Part model, mm, in its own coordinate system. A direction names the side the tool comes from. Round coordinates to 2 decimals unless told otherwise and drop trailing zeros. Order: outer loops, then holes, each group sorted by start corner. A loop starts at its lowest first (then second) coordinate and runs counter-clockwise, first axis right, second up. Notation, with made-up numbers: (69, -32) - (90, -32) arc R20 cw to (90, -28) - close; hole circle Ø8 at (4, 62.25). An arc over 180 degrees is marked (long way). Answer as a JSON object with one key per item and string values.
```python
from build123d import *

# Parameters (mm, degrees)
F0_R     = 12.7
F1_DEPTH = 58.42
F2_DEPTH = 19.05
F3_DEPTH = 19.05
F4_R     = 6.35
F5_DEPTH = 38.1
F6_R     = 3.302
F7_R     = 5.08
F8_R     = 7.874
F4_W     = 44.704
F4_H     = 20.4216
F4_W_2   = 6.096
F9_DEPTH = 38.1


# Not quite as in the source:
# - a feature names something its author has since deleted; it is built from what else it names


with BuildPart() as f1:
    # F0 (on Front) → F1 (new body)
    with BuildSketch(Plane.XZ):
        Polygon((85.852, 22.352), (91.8464, 0), (117.2464, 0), (117.2464, 22.352), align=None)
        with BuildLine():
            ThreePointArc((22.352, 22.352), (15.8052507731, 6.5467492269), (0, 0))
            Line((0, 0), (91.8464, 0))
            Line((91.8464, 0), (85.852, 22.352))
            Line((85.852, 22.352), (22.352, 22.352))
        make_face()
        Polygon((117.2464, 22.352), (117.2464, 0), (194.2084, 0), (194.2084, 22.352), (150.0886, 22.352), align=None)
        with BuildLine():
            ThreePointArc((22.352, 22.352), (-15.8052507731, 38.1572507731), (0, 0))
            ThreePointArc((0, 0), (15.8052507731, 6.5467492269), (22.352, 22.352))
        make_face()
        with Locations((0, 22.352)):
            Circle(F0_R, mode=Mode.SUBTRACT)
    extrude(amount=-F1_DEPTH)

    # F0 (on Front) → F2 (cut)
    with BuildSketch(Plane.XZ):
        Polygon((85.852, 22.352), (91.8464, 0), (117.2464, 0), (117.2464, 22.352), align=None)
    extrude(amount=-F2_DEPTH, mode=Mode.SUBTRACT)

    # F0 (on Front) → F3 (join)
    with BuildSketch(Plane.XZ):
        with BuildLine():
            ThreePointArc((131.0386, 57.15), (127.4644153616, 38.4343576341), (117.2464, 22.352))
            Line((117.2464, 22.352), (150.0886, 22.352))
            Line((150.0886, 22.352), (150.0886, 57.15))
            Line((150.0886, 57.15), (131.0386, 57.15))
        make_face()
    extrude(amount=-F3_DEPTH)

    # F4 (on face) → F5 (cut, symmetric)
    with BuildSketch(Plane.XY.offset(22.352)):
        with Locations((155.3464, 36.068)):
            Circle(F4_R)
    extrude(amount=F5_DEPTH, both=True, mode=Mode.SUBTRACT)

    # F6
    f6_edges = [f1.edges().sort_by_distance(p)[0] for p in [
        (22.352, 29.21, 22.352),
        (150.0886, 9.525, 22.352),
    ]]
    fillet(f6_edges, radius=F6_R)

    # F7
    f7_edges = [f1.edges().sort_by_distance(p)[0] for p in [
        (150.0886, 9.525, 57.15),
    ]]
    fillet(f7_edges, radius=F7_R)

    # F8
    f8_edges = [f1.edges().sort_by_distance(p)[0] for p in [
        (194.2084, 29.21, 22.352),
    ]]
    fillet(f8_edges, radius=F8_R)

    # F4 (on face) → F9 (cut, symmetric)
    with BuildSketch(Plane.XY.offset(22.352)):
        with Locations((0, 29.21)):
            Rectangle(F4_W, F4_H)
        with Locations((25.4, 29.21)):
            Rectangle(F4_W_2, F4_H)
        with Locations((155.3464, 36.068)):
            Circle(F4_R)
    extrude(amount=F9_DEPTH, both=True, mode=Mode.SUBTRACT)


solid = f1.part
```
Item 1: Two-plate mould, pull along X, no slides. Class faces 1 (the flat face through (28.448, 29, 11)), 2 (the cylindrical face through (161.4, 37.98, 11.33)), 3 (the flat face through (84, 58.42, 13)): pulls with the +X half, pulls with the -X half, needs draft (parallel to the pull), parting line crosses it, or undercut.
Taken from the geometry:
{"face 1": "pulls with the -X half", "face 2": "undercut", "face 3": "needs draft"}
Item 2: Cut at B-B (z = 20.5). Write the cut outline in (x, y), plus the area to 3 significant figures.
Taken from the geometry:
{"outline": "(-22.28, 0) - (-12.56, 0) - (-12.56, 19) - (-22.28, 19) - close; (-22.28, 39.42) - (-12.56, 39.42) - (-12.56, 58.42) - (-22.28, 58.42) - close; (12.56, 0) - (86.35, 0) - (86.35, 19.05) - (117.25, 19.05) - (117.25, 0) - (191.41, 0) - (191.41, 58.42) - (12.56, 58.42) - (12.56, 39.42) - (28.45, 39.42) - (28.45, 19) - (12.56, 19) - close; hole circle Ø12.7 at (155.35, 36.07)", "area": "9,780 mm2"}
Item 3: Probe L1, parallel to Y at x = -2.5, z = 42; L2, parallel to Z at x = 0, y = 54; L3, parallel to X at y = 8.5, z = 28.5. List the from-to ranges inside material, lowest first. Write a range as from..to.
Taken from the geometry:
{"L1": "0..19, 39.42..58.42", "L2": "0..9.65, 35.05..44.7", "L3": "-21.49..-11.11, 11.11..21.49, 122.19..150.09"}
Item 4: Cut at C-C (y = 34). Write the cut outline in (x, z).
Taken from the geometry:
{"outline": "(28.45, 0) - (149.34, 0) - (149.34, 22.35) - (28.45, 22.35) - close; (161.35, 0) - (194.21, 0) - (194.21, 14.48) arc R7.87 ccw to (186.33, 22.35) - (161.35, 22.35) - close"}
Item 5: Tool access for faces 4 (the flat face through (101, 19.05, 11)), 5 (the flat face through (150.089, 9, 39)), 6 (the flat face through (139, 19.05, 40)), 7 (the flat face through (107, 35, 22.352)): list every direction of +Z, -Z, +X, -X, +Y, -Y with a clear straight run to the whole face (end or side of a thin tool).
Taken from the geometry:
{"face 4": "+Z, -Y", "face 5": "+Z, +X, +Y, -Y", "face 6": "+Z, +X, -X, +Y", "face 7": "+Z, +Y"}
Item 6: Drop flat-ended pins along their axis: P1, Ø1, axis at x = 102, y = 26, coming from the -Z side; P2, Ø6, axis at x = 172.5, y = 23.5, coming from the +Z side; P3, Ø22.5, axis at y = 24.5, z = 8.5, coming from the -X side; P4, Ø5, axis at y = 15.5, z = 47, coming from the +X side. Give the stop position or say it passes through.
Taken from the geometry:
{"P1": "z = 0", "P2": "z = 22.35", "P3": "x = -21.98", "P4": "x = 150.09"}
Item 7: Cut at A-A (y = 11). Write the cut outline in (x, z).
Taken from the geometry:
{"outline": "(0, 0) - (91.85, 0) - (85.85, 22.35) - (25.44, 22.35) arc R3.3 cw to (22.17, 25.23) arc R22.35 ccw (long way) to start; (117.25, 0) - (194.21, 0) - (194.21, 14.48) arc R7.87 ccw to (186.33, 22.35) - (153.39, 22.35) arc R3.3 cw to (150.09, 25.65) - (150.09, 52.07) arc R5.08 ccw to (145.01, 57.15) - (131.04, 57.15) arc R50.8 cw to (117.25, 22.35) - close; hole circle Ø25.4 at (0, 22.35)"}
Item 8: Cut at D-D (x = 111). Write the cut outline in (y, z), plus the area to 3 significant figures.
Taken from the geometry:
{"outline": "(19.05, 0) - (58.42, 0) - (58.42, 22.35) - (19.05, 22.35) - close", "area": "880 mm2"}
